```python
from build123d import *

# Parameters (mm, degrees)
F1_DEPTH = 25.4
F2_W     = 16.863502562
F2_H     = 14.0826925635
F3_DEPTH = 25.4


with BuildPart() as f1:
    # F0 (on Front) → F1 (new body, symmetric)
    with BuildSketch(Plane.XZ):
        Polygon((0, 48.207629472), (0, 0), (70.2951550484, 0), (70.2951550484, 48.207629472), (53.4316524863, 48.207629472), (53.4316524863, 28.4113399684), (16.5885612369, 28.4113399684), (16.5885612369, 48.207629472), align=None)
    extrude(amount=F1_DEPTH, both=True)

    # F2 (on face) → F3 (cut)
    with BuildSketch(Plane.XY.offset(48.207629472)):
        with Locations((61.8634037673, 0.0867024064)):
            Rectangle(F2_W, F2_H)
    extrude(amount=-F3_DEPTH, mode=Mode.SUBTRACT)


solid = f1.part
```
Input: part model. Units: mm. Frame: model coordinates. A direction names the side the tool comes from. Coordinates: 2 decimals unless noted, no trailing zeros. Loops run counter-clockwise (first coordinate to the right, second up) from the corner with the lowest first, then second, coordinate; pieces in that order, holes last.
Q1. Section A-A, the plane z = 34.5. Return the cut outline in (x, y).
Results are:
outline: (0, -25.4) - (16.59, -25.4) - (16.59, 25.4) - (0, 25.4) - close; (53.43, -25.4) - (70.3, -25.4) - (70.3, -6.95) - (53.43, -6.95) - close; (53.43, 7.13) - (70.3, 7.13) - (70.3, 25.4) - (53.43, 25.4) - close
Q2. Section C-C, the plane y = -9. Return the cut outline in (x, z).
Results are:
outline: (0, 0) - (70.3, 0) - (70.3, 48.21) - (53.43, 48.21) - (53.43, 28.41) - (16.59, 28.41) - (16.59, 48.21) - (0, 48.21) - close
Q3. Line query: line 1 along X through (y, z) = (18, 34.5); line 2 along Z through (x, y) = (34.5, 21); line 3 along Y through (x, z) = (61.5, 40). Output: solid intervals per line, ascending.
Results are:
line 1: x = 0 to 16.59, 53.43 to 70.3
line 2: z = 0 to 28.41
line 3: y = -25.4 to -6.95, 7.13 to 25.4
Q4. Section D-D, the plane x = 48. Return the cut outline in (y, z), and give its area (3 significant figures).
Results are:
outline: (-25.4, 0) - (25.4, 0) - (25.4, 28.41) - (-25.4, 28.41) - close
area: 1,440 mm2
Q5. Contact query for flat-ended pins moving along their axis: pin 1 (1.7 mm diameter, centred on y = -2, z = 27, fed in from +X); pin 2 (7 mm diameter, centred on x = 65, y = -3, fed in from +Z). Output: stop coordinate, or through.
Results are:
pin 1: stops at x = 53.43
pin 2: stops at z = 22.81
Q6. Set-up query: faces 5 (the flat face through (35, -25.4, 19)), 6 (the flat face through (62, 0, 22.808)), 7 (the flat face through (16.589, 0, 38)). Return all of +Z, -Z, +X, -X, +Y, -Y with unobstructed straight access to the full face (end or side cutting, diameter ignored); none if empty.
Results are:
face 5: +Z, -Z, +X, -X, -Y
face 6: +Z, +X
face 7: +Z, +Y, -Y
Q7. Section B-B, the plane x = 63. Return the cut outline in (y, z).
Results are:
outline: (-25.4, 0) - (25.4, 0) - (25.4, 48.21) - (7.13, 48.21) - (7.13, 22.81) - (-6.95, 22.81) - (-6.95, 48.21) - (-25.4, 48.21) - close
Q8. Mould query, pull axis X, two halves, no side actions, for faces 1 (the flat face through (35, 25.4, 19)), 2 (the flat face through (0, 0, 24)), 3 (the flat face through (53.432, 0, 26)), 4 (the flat face through (53.432, -16, 38)). Classes: +X half, -X half, draft (parallel to the pull), parting line (faces both ways), or undercut.
Results are:
face 1: draft
face 2: -X half
face 3: +X half
face 4: undercut
